Geometry: see drawing. Coordinates: mm, zero at the bounding-box minimum. Give positions to 0.01 mm unless a question says otherwise; leave off trailing zeros. Order: outer loops, then holes, each group sorted by start corner. A loop starts at its lowest first (then second) coordinate and runs counter-clockwise, first axis right, second up. Notation, with made-up numbers: (-39.75, 45.25) - (7.25, 45.25) arc R20 cw to (7.25, 52.25) - close; hole circle Ø10 at (-27.5, 88.5). An arc over 180 degrees is marked (long way). Put each result on its own line as item: value. Start each with the question number.
1. First-contact query: P1, Ø0.8, axis at y = 1, z = 33, coming from the +X side. Flat tip, straight axial feed; report the tip coordinate or a pass-through.
2. Section A-A on z = 25.4. Return the cut outline in (x, y), plus the area to 3 significant figures.
3. Section C-C on z = 11. Return the cut outline in (x, y).
4. Ray query, line 1 along X through (y, z) = (2.25, 36.5). Return the intervals inside material, ascending. Write a range as from..to.
5. Section B-B on y = 1.27. Return the cut outline in (x, z).
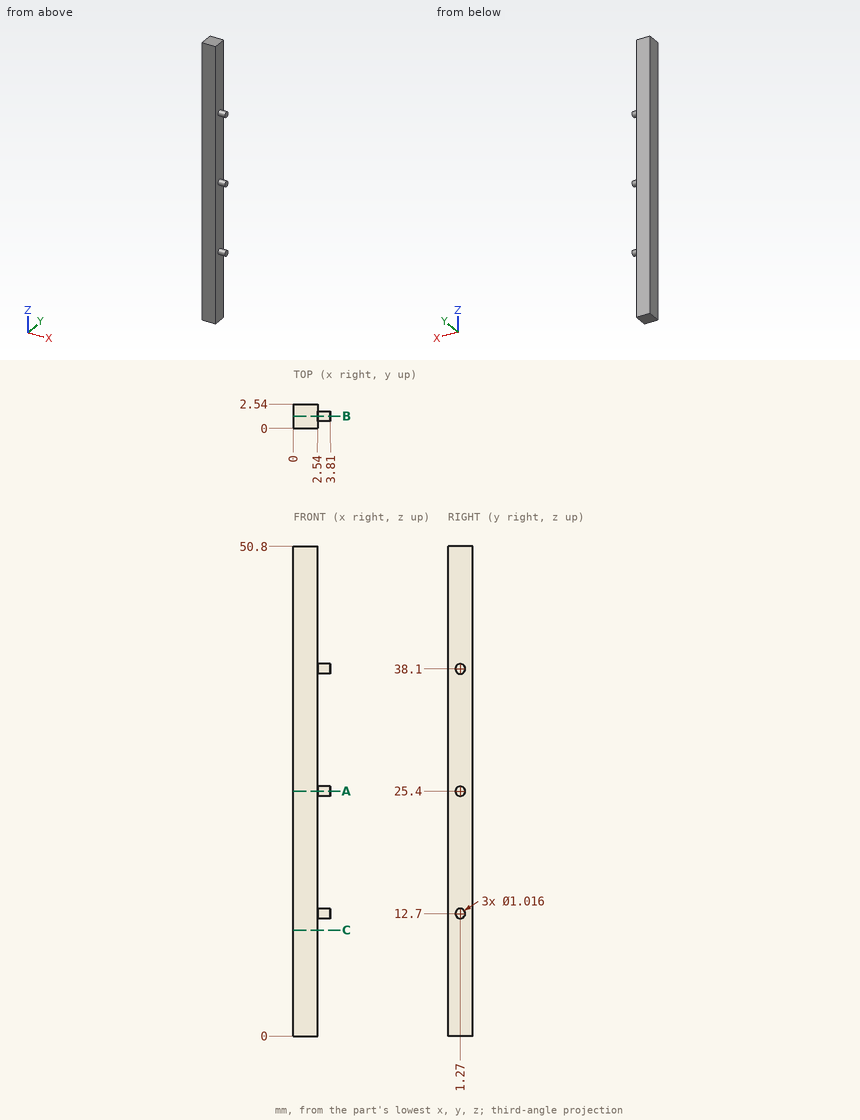
Resolved:
1. P1: x = 2.54
2. outline: (0, 0) - (2.54, 0) - (2.54, 0.76) - (3.81, 0.76) - (3.81, 1.78) - (2.54, 1.78) - (2.54, 2.54) - (0, 2.54) - close
2. area: 7.74 mm^2
3. outline: (0, 0) - (2.54, 0) - (2.54, 2.54) - (0, 2.54) - close
4. line 1: 0..2.54
5. outline: (0, 0) - (2.54, 0) - (2.54, 12.19) - (3.81, 12.19) - (3.81, 13.21) - (2.54, 13.21) - (2.54, 24.89) - (3.81, 24.89) - (3.81, 25.91) - (2.54, 25.91) - (2.54, 37.59) - (3.81, 37.59) - (3.81, 38.61) - (2.54, 38.61) - (2.54, 50.8) - (0, 50.8) - close
